Can you work these out from the model? Positions are in its coordinate system, mm. A direction names the side the tool comes from. Coordinates: 2 decimals unless noted, no trailing zeros. Order: outer loops, then holes, each group sorted by start corner. A loop starts at its lowest first (then second) coordinate and runs counter-clockwise, first axis right, second up. Notation, with made-up numbers: (23, 26.5) - (75, 26.5) arc R17 cw to (75, 34.5) - close; hole circle Ø9 at (27, 6). An arc over 180 degrees is marked (long way). Use a Markdown table: item, result. Add a question column.
(1) I want a section at D-D (y = -9). List the corners of the cut face in (x, z) for me.
(2) I want a section at B-B (y = -44). List the corners of the cut face in (x, z) for me, and give its area (3 significant figures).
(3) If I drill on L1, parallel to Z at x = 11.5, y = -1.4; L2, parallel to X at y = -1, z = -11; L3, parallel to Z at x = -11, y = -1, over which ranges is the centre line in solid material (lowest first)? Write a range as [from, to].
(4) We'd pull the mould along Z, two halves only. Please class faces 3 (the cylindrical face through (-17.986, -42.81, -12.934)), 4 (the flat face through (-17, -26, 0)), 5 (the flat face through (-6.2, -2.7, -17)), 6 (the cylindrical face through (-17.99, -11.81, 11.11)): pulls with the +Z half, pulls with the -Z half, needs draft (parallel to the pull), parting line crosses it, or undercut.
(5) I want a section at A-A (x = -11.5). List the corners of the cut face in (y, z) for me, and give its area (3 significant figures).
(6) On a 3-axis mill with a long thin cutter (end or side, diameter ignored), from which of +Z, -Z, +X, -X, +Y, -Y can I reach the whole of each face in a straight line? I mean faces 1 (the cylindrical face through (-12.974, -1.479, -10.148)), 2 (the flat face through (0, -3, 0)). Say none if no direction works.
(7) I want a section at C-C (z = -4). List the corners of the cut face in (x, y) for me.
(8) For pin 1 Ø5 at (x, z) = (-11.5, -11.5) entering from -Y; pin 2 Ø1.8 at (y, z) = (-13, 12.02) entering from +X; pin 3 Ø5 at (y, z) = (-42.5, -2.5) entering from +X; pin 4 Ø1 at (x, z) = (-15, 5) entering from +Y, each with a flat end and sliding along its axis, tell me the tip position at first contact or that it passes through.
```python
from build123d import *

# Parameters (mm, degrees)
F0_W     = 34
F0_H     = 34
F0_R     = 2
F1_DEPTH = 3
F2_R     = 1.5
F3_DEPTH = 2


with BuildPart() as f1:
    # F0 (on Front) → F1 (new body)
    with BuildSketch(Plane.XZ):
        Rectangle(F0_W, F0_H)
        with Locations((-11.5, -11.5)):
            Circle(F0_R, mode=Mode.SUBTRACT)
        with Locations((11.5, -11.5)):
            Circle(F0_R, mode=Mode.SUBTRACT)
        with Locations((-11.5, 11.5)):
            Circle(F0_R, mode=Mode.SUBTRACT)
        with Locations((11.5, 11.5)):
            Circle(F0_R, mode=Mode.SUBTRACT)
    extrude(amount=F1_DEPTH)

    # F2 (on face) → F3 (join)
    with BuildSketch(Plane(origin=(-17, 0, 0), x_dir=(0, -1, 0), z_dir=(-1, 0, 0))):
        Polygon((28.5, 17), (0, 17), (0, -17), (28.5, -17), (28.5, 0), align=None)
        with Locations((13, -12.021406)):
            Circle(F2_R, mode=Mode.SUBTRACT)
        with Locations((13, 12.021406)):
            Circle(F2_R, mode=Mode.SUBTRACT)
        Polygon((50, 17), (28.5, 17), (28.5, 0), (28.5, -17), (50, -17), align=None)
        with Locations((44, -12.021406)):
            Circle(F2_R, mode=Mode.SUBTRACT)
        with Locations((44, 12.021406)):
            Circle(F2_R, mode=Mode.SUBTRACT)
    extrude(amount=F3_DEPTH)


solid = f1.part
```
Answers follow:
| question | item | result |
|---|---|---|
| 1 | outline | (-19, -17) - (-17, -17) - (-17, 17) - (-19, 17) - close |
| 2 | outline | (-19, -17) - (-17, -17) - (-17, -13.52) - (-19, -13.52) - close; (-19, -10.52) - (-17, -10.52) - (-17, 10.52) - (-19, 10.52) - close; (-19, 13.52) - (-17, 13.52) - (-17, 17) - (-19, 17) - close |
| 2 | area | 56.0 mm² |
| 3 | L1 | z = [-17, -13.5], [-9.5, 9.5], [13.5, 17] |
| 3 | L2 | x = [-19, -13.44], [-9.56, 9.56], [13.44, 17] |
| 3 | L3 | z = [-17, -13.44], [-9.56, 9.56], [13.44, 17] |
| 4 | face 3 | undercut |
| 4 | face 4 | needs draft |
| 4 | face 5 | pulls with the -Z half |
| 4 | face 6 | undercut |
| 5 | outline | (-3, -17) - (0, -17) - (0, -13.5) - (-3, -13.5) - close; (-3, -9.5) - (0, -9.5) - (0, 9.5) - (-3, 9.5) - close; (-3, 13.5) - (0, 13.5) - (0, 17) - (-3, 17) - close |
| 5 | area | 78.0 mm² |
| 6 | face 1 | +Y, -Y |
| 6 | face 2 | +Z, -Z, +X, -Y |
| 7 | outline | (-19, -50) - (-17, -50) - (-17, -3) - (17, -3) - (17, 0) - (-19, 0) - close |
| 8 | pin 1 | stops at y = -3 |
| 8 | pin 2 | passes through |
| 8 | pin 3 | stops at x = -17 |
| 8 | pin 4 | stops at y = 0 |
